Here's the drawing with two shaded views (mm, measured from the low corner). I have some questions. A direction names the side the tool comes from. Coordinates: 2 decimals unless noted, no trailing zeros. Write each loop counter-clockwise with the first axis right and the second up, starting at its lowest first coordinate (ties: lowest second). Pieces come first, ordered by that corner, then holes.
Item 1: Which directions (+Z, -Z, +X, -X, +Y, -Y) give clear straight access to the entire face, cutting with the end or side of a thin tool? Please do the marked faces 1 and 2.
Item 2: For P1, Ø6, axis at x = 112.5, z = 7.5, coming from the -Y side (1 decimal); P2, Ø3, axis at y = 88.5, z = 15.5, coming from the -X side; P3, Ø10, axis at y = 127.5, z = 13.5, coming from the +X side, each with a flat end and sliding along its axis, tell me the tip position at first contact or that it passes through.
Item 3: I want a section at B-B on x = 147. Please give me the cut outline in (y, z) (1 decimal).
Item 4: I want a section at A-A on z = 15. Please give me the cut outline in (x, y) (1 decimal), then the cut area to 3 significant figures.
Item 5: If I drill on probe 1 along Y at (x, z) = (257, 13.5) (1 decimal); probe 2 along Z at (x, y) = (138, 158); probe 3 along Y at (x, z) = (103.5, 15.75) (1 decimal), over which ranges is the centre line in solid material (lowest first)?
Item 6: I want a section at D-D on x = 74. Please give me the cut outline in (y, z) (1 decimal), then the cut area to 3 significant figures.
Item 7: I want a section at C-C on y = 67.5. Please give me the cut outline in (x, z).
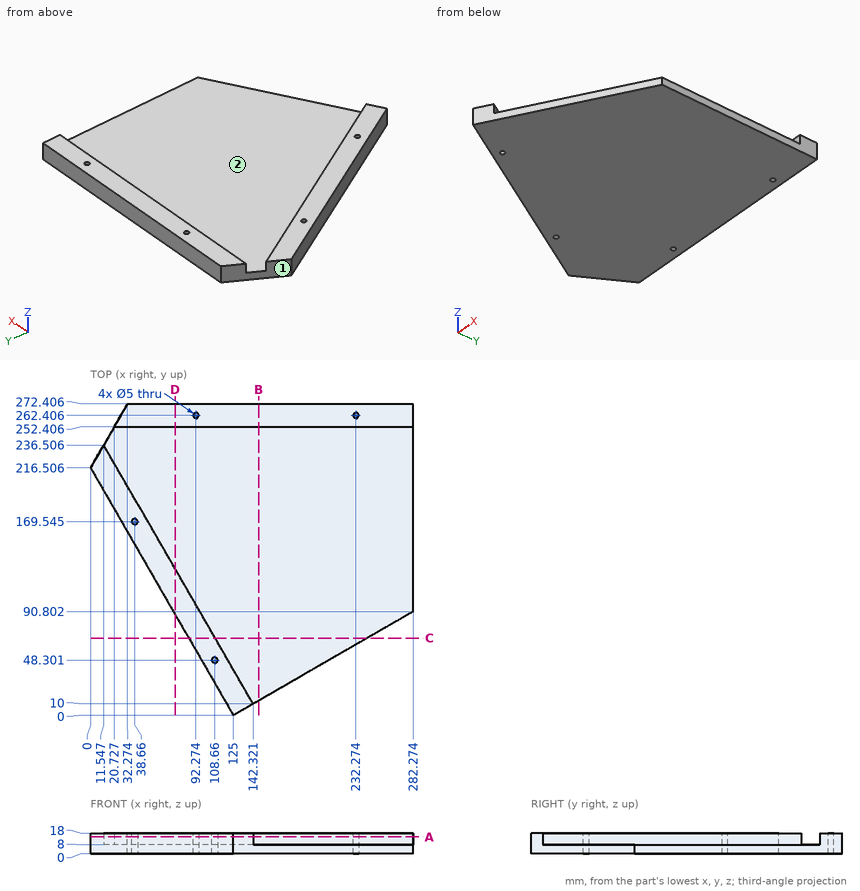
Response values:
1. face 1: +Z, -Z, -X, +Y
1. face 2: +Z, +X
2. P1: stops at y = 16.5
2. P2: stops at x = 73.04
2. P3: stops at x = 77.37
3. outline: (12.7, 0) - (272.4, 0) - (272.4, 18) - (252.4, 18) - (252.4, 8) - (12.7, 8) - close
4. outline: (0, 216.5) - (125, 0) - (142.3, 10) - (11.5, 236.5) - close; (20.7, 252.4) - (282.3, 252.4) - (282.3, 272.4) - (32.3, 272.4) - close; hole circle Ø5 at (38.7, 169.5); hole circle Ø5 at (92.3, 262.4); hole circle Ø5 at (108.7, 48.3); hole circle Ø5 at (232.3, 262.4)
4. area: 10,200 mm2
5. probe 1: y = 252.4 to 272.4
5. probe 2: z = 0 to 8
5. probe 3: y = 37.2 to 77.2, 252.4 to 272.4
6. outline: (88.3, 0) - (272.4, 0) - (272.4, 18) - (252.4, 18) - (252.4, 8) - (128.3, 8) - (128.3, 18) - (88.3, 18) - close
6. area: 2,070 mm2
7. outline: (86.03, 0) - (241.91, 0) - (241.91, 8) - (109.12, 8) - (109.12, 18) - (86.03, 18) - close
